Part model, mm, in its own coordinate system. Face numbers are marked on the shaded views. A direction names the side the tool comes from. Round coordinates to 2 decimals unless told otherwise and drop trailing zeros. Write each loop counter-clockwise with the first axis right and the second up, starting at its lowest first coordinate (ties: lowest second). Pieces come first, ordered by that corner, then holes.
```python
from build123d import *

# Parameters (mm, degrees)
SKETCH1_R           = 3.4798
BOSS_EXTRUDE1_DEPTH = 8.509
SKETCH2_R           = 1.0414
BOSS_EXTRUDE2_DEPTH = 23.749
SKETCH3_OUTSIDE_W   = 15.706
SKETCH3_OUTSIDE_H   = 15.706
CUT_EXTRUDE1_DEPTH  = 8.509


with BuildPart() as part:
    # Sketch1 → Boss-Extrude1 (new body)
    with BuildSketch(Plane(origin=(0, 0, 0), x_dir=(1, 0, 0), z_dir=(0, 1, 0))):
        with Locations(Location((0, 0, 0), (0, 0, 270))):
            Circle(SKETCH1_R)
    extrude(amount=BOSS_EXTRUDE1_DEPTH)

    # Sketch2 → Boss-Extrude2 (add)
    with BuildSketch(Plane.XZ):
        with Locations(Location((0, 0, 0), (0, 0, 90))):
            Circle(SKETCH2_R)
    extrude(amount=BOSS_EXTRUDE2_DEPTH)

    # Sketch3 outside → Cut-Extrude1 (cut)
    with BuildSketch(Plane(origin=(0, 8.509, 0), x_dir=(1, 0, 0), z_dir=(0, 1, 0))):
        Rectangle(SKETCH3_OUTSIDE_W, SKETCH3_OUTSIDE_H)
        with BuildLine():
            Line((-2.612467483, 2.2987), (2.612467483, 2.2987))
            ThreePointArc((2.612467483, 2.2987), (3.4798, 0), (2.612467483, -2.2987))
            Line((2.612467483, -2.2987), (-2.612467483, -2.2987))
            ThreePointArc((-2.612467483, -2.2987), (-3.4798, 0), (-2.612467483, 2.2987))
        make_face(mode=Mode.SUBTRACT)
    extrude(amount=-CUT_EXTRUDE1_DEPTH, mode=Mode.SUBTRACT)


solid = part.part
```
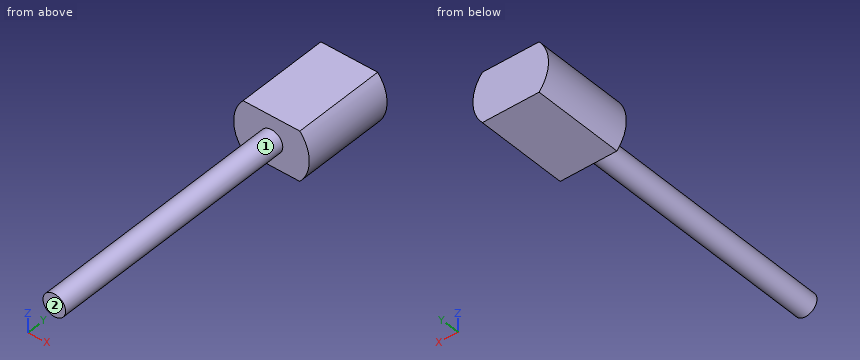
Q1. Drop flat-ended pins along their axis: pin 1 (1 mm diameter, centred on x = 2, y = -15.5, fed in from -Z); pin 2 (2 mm diameter, centred on y = -13, z = -1, fed in from -X). Give the stop position or say it passes through.
Values follow:
pin 1: passes through
pin 2: stops at x = -1.04
Q2. Which spindle directions (+Z, -Z, +X, -X, +Y, -Y) get a long thin tool onto all of the face, cutting with end or side? Do the marked faces 1 and 2. Say none if no direction does.
Values follow:
face 1: -Y
face 2: +Z, -Z, +X, -X, -Y
Q3. Cut at B-B on z = 0. Write the cut outline in (x, y).
Values follow:
outline: (-3.48, 0) - (-1.04, 0) - (-1.04, -23.75) - (1.04, -23.75) - (1.04, 0) - (3.48, 0) - (3.48, 8.51) - (-3.48, 8.51) - close
Q4. Cut at D-D on y = 5. Write the cut outline in (x, z).
Values follow:
outline: (-2.61, -2.3) - (2.61, -2.3) arc R3.48 ccw to (2.61, 2.3) - (-2.61, 2.3) arc R3.48 ccw to start
Q5. Cut at C-C on y = -15.5. Write the cut outline in (x, z).
Values follow:
outline: circle Ø2.08 at (0, 0)
Q6. Cut at A-A on x = 0. Write the cut outline in (y, z), plus the area to 3 significant figures.
Values follow:
outline: (-23.75, -1.04) - (0, -1.04) - (0, -2.3) - (8.51, -2.3) - (8.51, 2.3) - (0, 2.3) - (0, 1.04) - (-23.75, 1.04) - close
area: 88.6 mm2
Q7. Wall check: L1, parallel to Y at x = -3, z = -0.25; L2, parallel to X at y = -8, z = -0.1; L3, parallel to X at y = 2.5, z = -0.1. Give the ranges that are in metal, low to high.
Values follow:
L1: y = 0 to 8.51
L2: x = -1.04 to 1.04
L3: x = -3.48 to 3.48
